```python
from build123d import *

# Parameters (mm, degrees)
F1_DEPTH = 17
F2_R     = 11.691727
F3_DEPTH = 14
F4_R     = 4.624372
F4_R_2   = 4.285959
F4_R_3   = 4.957168
F5_DEPTH = 25
F7_DEPTH = 0.5


with BuildPart() as f1:
    # F0 (on Front) → F1 (new body)
    with BuildSketch(Plane.XZ):
        with BuildLine():
            Line((-40, -27.427316), (-28.084865, -40.25))
            Line((-28.084865, -40.25), (29.84, -40.25))
            ThreePointArc((29.84, -40.25), (40.960822, -33.683297), (40.581307, -20.773989))
            ThreePointArc((40.581307, -20.773989), (39.938227, -20.134126), (39.080779, -19.837887))
            ThreePointArc((39.080779, -19.837887), (-0.21216, 0.836167), (-14.717551, 42.799785))
            ThreePointArc((-14.717551, 42.799785), (-15.264908, 44.170434), (-16.654855, 44.666745))
            ThreePointArc((-16.654855, 44.666745), (-33.272886, 36.568692), (-40, 19.35))
            Line((-40, 19.35), (-40, -27.427316))
        make_face()
    extrude(amount=F1_DEPTH)

    # F2 (on face) → F3 (cut)
    with BuildSketch(Plane.XZ.offset(17)):
        with Locations((-5.678192, -10.890958)):
            Circle(F2_R)
    extrude(amount=-F3_DEPTH, mode=Mode.SUBTRACT)

    # F4 (on face) → F5 (cut)
    with BuildSketch(Plane.XZ.offset(17)):
        with Locations((-20.199468, 4.74734)):
            Circle(F4_R)
        with Locations((-30.25266, 29.135641)):
            Circle(F4_R_2)
        with Locations((9.587764, -27.087769)):
            Circle(F4_R_3)
    extrude(amount=-F5_DEPTH, mode=Mode.SUBTRACT)

    # F6 (on face) → F7 (cut)
    with BuildSketch(Plane(origin=(0, 0, 0), x_dir=(-1, 0, 0), z_dir=(0, 1, 0))):
        with BuildLine():
            ThreePointArc((-37.470929, -34.75125), (10.350502, -10.34579), (29.774692, 39.706348))
            Line((29.774692, 39.706348), (29.774692, 45.691768))
            ThreePointArc((29.774692, 45.691768), (23.636454, 48.375894), (17.059354, 49.650356))
            Line((17.059354, 49.650356), (9.722393, 42.579803))
            ThreePointArc((9.722393, 42.579803), (-3.580862, 4.093924), (-39.617395, -14.866766))
            Line((-39.617395, -14.866766), (-44.810167, -18.106268))
            ThreePointArc((-44.810167, -18.106268), (-47.539999, -27.55), (-44.810167, -36.993732))
            Line((-44.810167, -36.993732), (-37.470929, -34.75125))
        make_face()
    extrude(amount=-F7_DEPTH, mode=Mode.SUBTRACT)


solid = f1.part
```
CAD build for the part. Positions are in the model's coordinates, mm. A direction names the side the tool comes from. Round coordinates to 2 decimals unless told otherwise and drop trailing zeros. Write each loop counter-clockwise with the first axis right and the second up, starting at its lowest first coordinate (ties: lowest second). Pieces come first, ordered by that corner, then holes. Notation, with made-up numbers: (79.25, 28.25) -> (122.25, 28.25) arc R23 ccw to (122.25, 36.25) -> close; hole circle Ø3 at (73, -5.5). An arc over 180 degrees is marked (long way). Answer in a Markdown table with one row per item. Add a question column.
Item 1: Saw through at C-C, the plane x = 35. Write the cut outline in (y, z), then the cut area to 3 significant figures.
Item 2: Mould opens along X. For faces 1 (the face through (0.205, -8.634, 0.355)), 2 (the face through (-34.126, -8.381, -33.749)), 3 (the face through (-17.36, -10.1, -10.38)) say: pulls with the +X half, pulls with the -X half, needs draft (parallel to the pull), parting line crosses it, or undercut.
Item 3: Which spindle directions (+Z, -Z, +X, -X, +Y, -Y) get a long thin tool onto all of the face, cutting with end or side? Do faces 4 (the face through (-18, -17, -7)), 5 (the face through (-6, -3, -11)), 6 (the face through (1, -0.5, -4)). Say none if no direction does.
Item 4: Saw through at B-B, the plane y = -10.5. Write the cut outline in (x, z), then the cut area to 3 significant figures.
Item 5: Saw through at A-A, the plane z = 32. Write the cut outline in (x, y), then the cut area to 3 significant figures.
Item 6: Drop flat-ended pins along their axis: pin 1 Ø6 at (y, z) = (-3.5, 36) entering from -X; pin 2 Ø4 at (y, z) = (-6.5, -13.5) entering from +X; pin 3 Ø15 at (x, z) = (-20.2, 4.75) entering from +Y; pin 4 Ø12 at (x, z) = (-17, 29) entering from +Y. Give the stop position or say it passes through.
Item 7: Saw through at D-D, the plane z = -4.5. Write the cut outline in (x, y).
Item 8: Drill centre lines: line 1 (X direction, y = -15, z = -27); line 2 (Y direction, x = 4, z = -11); line 3 (Z direction, x = -5.5, y = -4.75). Where is each one in solid material? Low to high. Write a range as from..to.
Findings below:
| question | item | result |
|---|---|---|
| 1 | outline | (-17, -39.15) -> (0, -39.15) -> (0, -34.44) -> (-0.5, -34.44) -> (-0.5, -19.26) -> (-17, -19.26) -> close |
| 1 | area | 331 mm^2 |
| 2 | face 1 | pulls with the +X half |
| 2 | face 2 | pulls with the -X half |
| 2 | face 3 | undercut |
| 3 | face 4 | +Z, -Z, +X, -X, -Y |
| 3 | face 5 | -Y |
| 3 | face 6 | +Z, +X, +Y |
| 4 | outline | (-40, -27.43) -> (-28.08, -40.25) -> (29.84, -40.25) arc R12.7 ccw to (40.58, -20.77) arc R2.03 ccw to (39.08, -19.84) arc R60.33 cw to (-14.72, 42.8) arc R1.79 ccw to (-16.65, 44.67) arc R25.4 ccw to (-40, 19.35) -> close; hole circle Ø8.57 at (-30.25, 29.14); hole circle Ø9.25 at (-20.2, 4.75); hole circle Ø23.38 at (-5.68, -10.89); hole circle Ø9.91 at (9.59, -27.09) |
| 4 | area | 3,190 mm^2 |
| 5 | outline | (-36.63, -17) -> (-33.44, -17) -> (-33.44, 0) -> (-36.63, 0) -> close; (-27.06, -17) -> (-14.22, -17) -> (-14.22, -0.5) -> (-27.06, -0.5) -> close |
| 5 | area | 266 mm^2 |
| 6 | pin 1 | stops at x = -36.02 |
| 6 | pin 2 | stops at x = 22.24 |
| 6 | pin 3 | stops at y = 0 |
| 6 | pin 4 | stops at y = -0.5 |
| 7 | outline | (-40, -17) -> (-15.47, -17) -> (-15.47, -3) -> (4.11, -3) -> (4.11, -17) -> (4.98, -17) -> (4.98, -0.5) -> (-15.12, -0.5) -> (-15.12, 0) -> (-40, 0) -> close |
| 8 | line 1 | x = -40..4.63, 14.54..42.53 |
| 8 | line 2 | y = -3..-0.5 |
| 8 | line 3 | z = -40.25..-22.58, 0.8..8 |
